Part print with two shaded views. Sizes in mm from the minimum x, y, z corner. A direction names the side the tool comes from. Round coordinates to 2 decimals unless told otherwise and drop trailing zeros. Loops run counter-clockwise (first coordinate to the right, second up) from the corner with the lowest first, then second, coordinate; pieces in that order, holes last.
(1) Cut at C-C on y = 5.75. List the corners of the cut face in (x, z), then the cut area to 3 significant figures.
(2) Cut at A-A on z = 2.2. List the corners of the cut face in (x, y), then the cut area to 3 significant figures.
(3) Probe probe 1 along Y at (x, z) = (4.75, 3.9); probe 2 along Y at (x, z) = (3.75, 5.3); probe 3 along Z at (x, y) = (2, 7.5). List the from-to ranges inside material, lowest first.
(4) Flat gauge pins, fed straight in: pin 1 (3 mm diameter, centred on y = 1, z = 3.5, fed in from -X); pin 2 (0.8 mm diameter, centred on x = 6, y = 5.5, fed in from +Z). Where does each tip first touch, or does it go through?
(5) Tool access for the marked faces 1 and 2: list every direction of +Z, -Z, +X, -X, +Y, -Y with a clear straight run to the whole face (end or side of a thin tool).
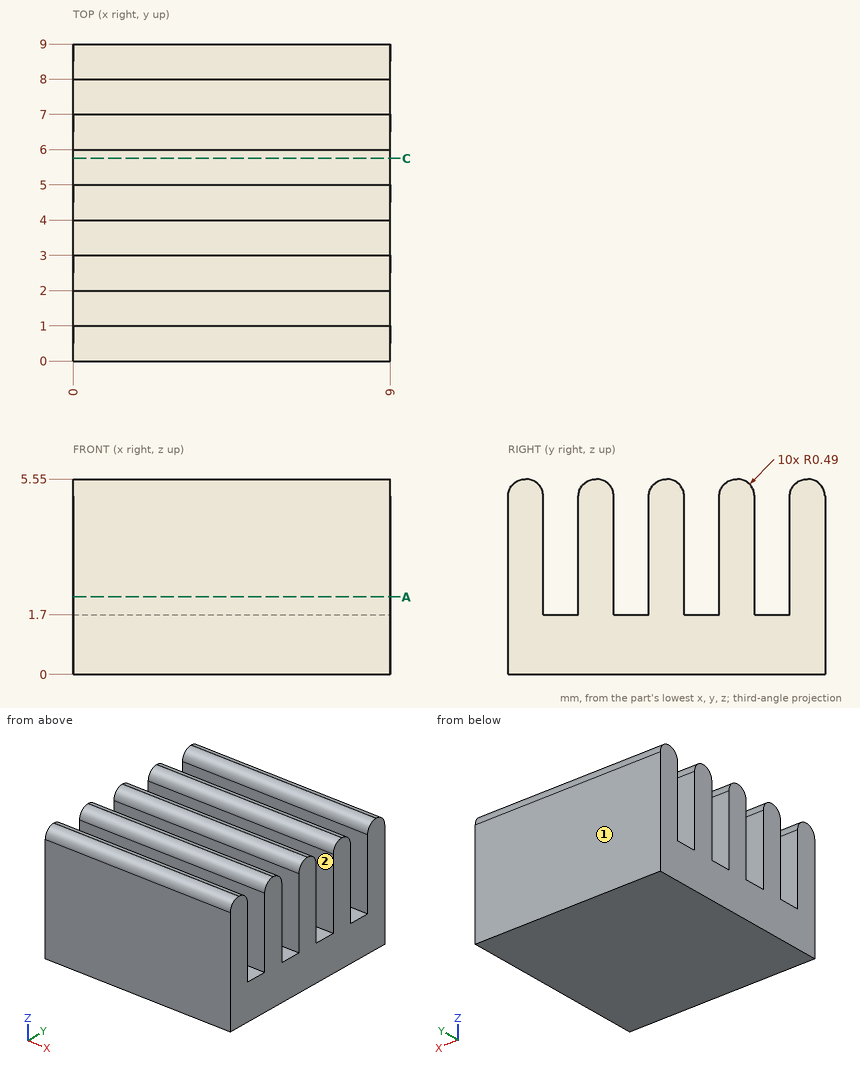
Final values:
1. outline: (0, 0) - (9, 0) - (9, 1.7) - (0, 1.7) - close
1. area: 15.3 mm2
2. outline: (0, 0) - (9, 0) - (9, 1) - (0, 1) - close; (0, 2) - (9, 2) - (9, 3) - (0, 3) - close; (0, 4) - (9, 4) - (9, 5) - (0, 5) - close; (0, 6) - (9, 6) - (9, 7) - (0, 7) - close; (0, 8) - (9, 8) - (9, 9) - (0, 9) - close
2. area: 45.0 mm2
3. probe 1: y = 0 to 1, 2 to 3, 4 to 5, 6 to 7, 8 to 9
3. probe 2: y = 0.06 to 0.94, 2.06 to 2.94, 4.06 to 4.94, 6.06 to 6.94, 8.06 to 8.94
3. probe 3: z = 0 to 1.7
4. pin 1: stops at x = 0
4. pin 2: stops at z = 1.7
5. face 1: +Z, -Z, +X, -X, +Y
5. face 2: +Z, +X, -X
